Input: part model. Units: mm. Frame: model coordinates. Coordinates: 2 decimals unless noted, no trailing zeros. Order: outer loops, then holes, each group sorted by start corner. A loop starts at its lowest first (then second) coordinate and runs counter-clockwise, first axis right, second up. Notation, with made-up numbers: (24.25, -28.5) -> (66.25, -28.5) arc R16 cw to (66.25, -7.5) -> close; hole circle Ø3 at (70.5, 72). An arc over 180 degrees is marked (long way). One line per question, with ' | ' between items.
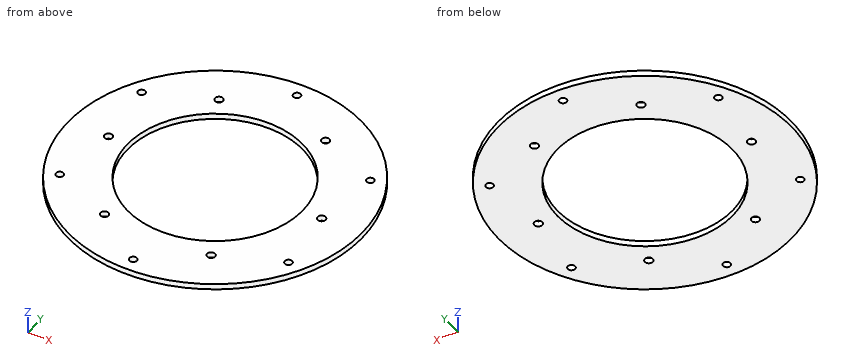
```python
from build123d import *

# Parameters (mm, degrees)
F0_R     = 129
F0_R_2   = 3.5
F0_R_3   = 3.25
F0_R_4   = 77
F1_DEPTH = 5


with BuildPart() as f1:
    # F0 (on Top) → F1 (new body)
    with BuildSketch(Plane.XY):
        Circle(F0_R)
        with Locations((-47, -81.406388)):
            Circle(F0_R_2, mode=Mode.SUBTRACT)
        with Locations((-100.89196, -58.25)):
            Circle(F0_R_3, mode=Mode.SUBTRACT)
        with Locations((0, -116.5)):
            Circle(F0_R_3, mode=Mode.SUBTRACT)
        with Locations((47, -81.406388)):
            Circle(F0_R_2, mode=Mode.SUBTRACT)
        with Locations((100.89196, -58.25)):
            Circle(F0_R_3, mode=Mode.SUBTRACT)
        with Locations((-94, 0)):
            Circle(F0_R_2, mode=Mode.SUBTRACT)
        with Locations((-100.89196, 58.25)):
            Circle(F0_R_3, mode=Mode.SUBTRACT)
        with Locations((-47, 81.406388)):
            Circle(F0_R_2, mode=Mode.SUBTRACT)
        Circle(F0_R_4, mode=Mode.SUBTRACT)
        with Locations((94, 0)):
            Circle(F0_R_2, mode=Mode.SUBTRACT)
        with Locations((100.89196, 58.25)):
            Circle(F0_R_3, mode=Mode.SUBTRACT)
        with Locations((47, 81.406388)):
            Circle(F0_R_2, mode=Mode.SUBTRACT)
        with Locations((0, 116.5)):
            Circle(F0_R_3, mode=Mode.SUBTRACT)
    extrude(amount=F1_DEPTH)


solid = f1.part
```
1. Cut plane A-A, the plane y = 116.5. Return loops of the section in (x, z).
Recorded:
outline: (-55.4, 0) -> (-3.25, 0) -> (-3.25, 5) -> (-55.4, 5) -> close; (3.25, 0) -> (55.4, 0) -> (55.4, 5) -> (3.25, 5) -> close
2. Pin query (flat end, axial travel): pin 1 Ø7.5 at (x, y) = (100.89, -58.25) entering from +Z; pin 2 Ø6.5 at (x, y) = (47, 81.41) entering from -Z; pin 3 Ø3 at (x, z) = (-65.5, 1.5) entering from +Y; pin 4 Ø2 at (y, z) = (-52.5, 2.5) entering from +X. Return the tip coordinate at first contact, or that it passes through.
Recorded:
pin 1: stops at z = 5 | pin 2: passes through | pin 3: stops at y = 112 | pin 4: stops at x = 118.27
3. Cut plane D-D, the plane x = -94. Return loops of the section in (y, z).
Recorded:
outline: (-88.35, 0) -> (-3.5, 0) -> (-3.5, 5) -> (-88.35, 5) -> close; (3.5, 0) -> (88.35, 0) -> (88.35, 5) -> (3.5, 5) -> close
4. Ray query, line 1 (Y direction, x = 0, z = 4.05); line 2 (Y direction, x = 47, z = 2); line 3 (X direction, y = 22.5, z = 4.5). Return the intervals inside material, ascending. Write a range as [from, to].
Recorded:
line 1: y = [-129, -119.75], [-113.25, -77], [77, 113.25], [119.75, 129] | line 2: y = [-120.13, -84.91], [-77.91, -60.99], [60.99, 77.91], [84.91, 120.13] | line 3: x = [-127.02, -73.64], [73.64, 127.02]
5. Cut plane B-B, the plane z = 3.35. State how many separate pieces and enclosed holes the cut face has, and give its area (3 significant figures).
Recorded:
separate pieces: 1 | enclosed holes: 13 | area: 33,200 mm^2
6. Cut plane C-C, the plane x = 47. Return loops of the section in (y, z), and give its area (3 significant figures).
Recorded:
outline: (-120.13, 0) -> (-84.91, 0) -> (-84.91, 5) -> (-120.13, 5) -> close; (-77.91, 0) -> (-60.99, 0) -> (-60.99, 5) -> (-77.91, 5) -> close; (60.99, 0) -> (77.91, 0) -> (77.91, 5) -> (60.99, 5) -> close; (84.91, 0) -> (120.13, 0) -> (120.13, 5) -> (84.91, 5) -> close | area: 521 mm^2
